Could you check a few things on this model? Use its own coordinates, in mm. A direction names the side the tool comes from. Round coordinates to 2 decimals unless told otherwise and drop trailing zeros. Write each loop counter-clockwise with the first axis right and the second up, starting at its lowest first coordinate (ties: lowest second). Pieces come first, ordered by that corner, then holes.
```python
from build123d import *

# Parameters (mm, degrees)
SKETCH1_W           = 12
SKETCH1_H           = 60
BOSS_EXTRUDE1_DEPTH = 4
SKETCH2_W           = 10
SKETCH2_H           = 5
BOSS_EXTRUDE2_DEPTH = 10
CUT_EXTRUDE1_REACH  = 63.123
SKETCH3_R           = 3
SKETCH6_W           = 20
SKETCH6_H           = 5
BOSS_EXTRUDE4_DEPTH = 2
CUT_EXTRUDE2_REACH  = 35.823
SKETCH13_W          = 5
SKETCH13_H          = 5
CUT_EXTRUDE3_REACH  = 35.823
SKETCH14_R          = 1.6
CUT_EXTRUDE4_REACH  = 36.583
SKETCH4_R           = 2


with BuildPart() as part:
    # Sketch1 → Boss-Extrude1 (new body)
    with BuildSketch(Plane(origin=(0, 0, 0), x_dir=(1, 0, 0), z_dir=(0, 1, 0))):
        Rectangle(SKETCH1_W, SKETCH1_H)
    extrude(amount=BOSS_EXTRUDE1_DEPTH)

    # Sketch2 → Boss-Extrude2 (add)
    with BuildSketch(Plane.XZ):
        with Locations((0, 27.5)):
            Rectangle(SKETCH2_W, SKETCH2_H)
    extrude(amount=BOSS_EXTRUDE2_DEPTH)

    # Sketch3 → Cut-Extrude1 (cut, up to next)
    with BuildSketch(Plane.XY.offset(30), mode=Mode.PRIVATE) as cut_extrude1_sk1:
        with Locations((0, -5.5)):
            Circle(SKETCH3_R)
    cut_extrude1_tool1 = extrude(cut_extrude1_sk1.sketch, amount=-CUT_EXTRUDE1_REACH, mode=Mode.PRIVATE) & part.part
    add(cut_extrude1_tool1.solids().sort_by_distance((0, -5.5, 30))[0], mode=Mode.SUBTRACT)

    # Sketch6 → Boss-Extrude4 (add)
    with BuildSketch(Plane(origin=(0, 0, 0), x_dir=(1, 0, 0), z_dir=(0, 1, 0))):
        with Locations((0, 27.5)):
            Rectangle(SKETCH6_W, SKETCH6_H)
    extrude(amount=BOSS_EXTRUDE4_DEPTH)

    # Sketch13 → Cut-Extrude2 (cut, up to next)
    with BuildSketch(Plane(origin=(0, 2, 0), x_dir=(1, 0, 0), z_dir=(0, 1, 0)), mode=Mode.PRIVATE) as cut_extrude2_sk1:
        with Locations((-7.5, 27.5)):
            Rectangle(SKETCH13_W, SKETCH13_H)
    cut_extrude2_tool1 = extrude(cut_extrude2_sk1.sketch, amount=CUT_EXTRUDE2_REACH, mode=Mode.PRIVATE) & part.part
    cut_extrude2 = cut_extrude2_tool1.solids().sort_by_distance((-7.5, 2, -27.5))[0]
    add(cut_extrude2, mode=Mode.SUBTRACT)

    # Sketch14 → Cut-Extrude3 (cut, up to next)
    with BuildSketch(Plane(origin=(0, 2, 0), x_dir=(1, 0, 0), z_dir=(0, 1, 0)), mode=Mode.PRIVATE) as cut_extrude3_sk1:
        with Locations(Location((-7.5, 27.5, 0), (0, 0, 270))):
            Circle(SKETCH14_R)
    cut_extrude3_tool1 = extrude(cut_extrude3_sk1.sketch, amount=-CUT_EXTRUDE3_REACH, mode=Mode.PRIVATE) & part.part
    cut_extrude3 = cut_extrude3_tool1.solids().sort_by_distance((-7.5, 2, -27.5))[0]
    add(cut_extrude3, mode=Mode.SUBTRACT)

    # Mirror1: Cut-Extrude2, Cut-Extrude3 across plane
    add(cut_extrude2.mirror(Plane(origin=(0, 0, 0), x_dir=(0, 0, 1), z_dir=(1, 0, 0))), mode=Mode.SUBTRACT)
    add(cut_extrude3.mirror(Plane(origin=(0, 0, 0), x_dir=(0, 0, 1), z_dir=(1, 0, 0))), mode=Mode.SUBTRACT)

    # Sketch4 → Cut-Extrude4 (cut, up to next)
    with BuildSketch(Plane(origin=(0, 4, 0), x_dir=(1, 0, 0), z_dir=(0, 1, 0)), mode=Mode.PRIVATE) as cut_extrude4_sk1:
        with Locations(Location((0, 0, 0), (0, 0, 270))):
            Circle(SKETCH4_R)
    cut_extrude4_tool1 = extrude(cut_extrude4_sk1.sketch, amount=-CUT_EXTRUDE4_REACH, mode=Mode.PRIVATE) & part.part
    add(cut_extrude4_tool1.solids().sort_by_distance((0, 4, 0))[0], mode=Mode.SUBTRACT)


solid = part.part
```
Q1. Imagine slicing it at C-C, the plane y = -5.5. Write out the boundary of the cut face in (x, z), then the cut area to 3 significant figures.
Q2. Imagine slicing it at A-A, the plane z = 0. Write out the boundary of the cut face in (x, y).
Q3. We'd pull the mould along X, two halves only. Please class faces 1 (the flat face through (-9, 2, -29)), 2 (the cylindrical face through (8.47, 1.01, -28.77)), 3 (the flat face through (10, 1, -27)): pulls with the +X half, pulls with the -X half, needs draft (parallel to the pull), parting line crosses it, or undercut.
Q4. On a 3-axis mill with a long thin cutter (end or side, diameter ignored), from which of +Z, -Z, +X, -X, +Y, -Y can I reach the whole of each face in a straight line? I mean faces 4 (the flat face through (6, 2, 3)), 5 (the flat face through (-5.5, 3, -25)), 6 (the flat face through (-8, 1, -25)). Say none if no direction works.
Q5. I'm going to push flat-ended pins straight in: pin 1 Ø10 at (x, z) = (1.5, 14) entering from -Y; pin 2 Ø2 at (x, y) = (-8.5, 1) entering from +Z; pin 3 Ø4.5 at (y, z) = (1.5, -6.5) entering from +X. Where does each tip first touch, or does it pass through?
Q6. Imagine slicing it at B-B, the plane x = 0. Write out the boundary of the cut face in (y, z).
Q7. Imagine slicing it at D-D, the plane z = -10. Write out the boundary of the cut face in (x, y), then the cut area to 3 significant figures.
Q8. If I drill on L1, parallel to X at y = 1.1, z = -27.5; L2, parallel to X at y = 3.1, z = 0; L3, parallel to Y at x = 0, z = 26.55, over which ranges is the centre line in solid material (lowest first)?
Results found:
1. outline: (-5, 25) - (-3, 25) - (-3, 30) - (-5, 30) - close; (3, 25) - (5, 25) - (5, 30) - (3, 30) - close
1. area: 20.0 mm2
2. outline: (-6, 0) - (-2, 0) - (-2, 4) - (-6, 4) - close; (2, 0) - (6, 0) - (6, 4) - (2, 4) - close
3. face 1: needs draft
3. face 2: undercut
3. face 3: pulls with the +X half
4. face 4: +Z, +X, +Y, -Y
4. face 5: -Z, -X, +Y
4. face 6: +Z, -X, +Y, -Y
5. pin 1: stops at y = 0
5. pin 2: stops at z = -25
5. pin 3: stops at x = 6
6. outline: (-10, 25) - (-8.5, 25) - (-8.5, 30) - (-10, 30) - close; (-2.5, 25) - (0, 25) - (0, 2) - (4, 2) - (4, 30) - (-2.5, 30) - close; (0, -30) - (4, -30) - (4, -2) - (0, -2) - close
7. outline: (-6, 0) - (6, 0) - (6, 4) - (-6, 4) - close
7. area: 48.0 mm2
8. L1: x = -10 to -9.1, -5.9 to 5.9, 9.1 to 10
8. L2: x = -6 to -2, 2 to 6
8. L3: y = -10 to -8.5, -2.5 to 4
